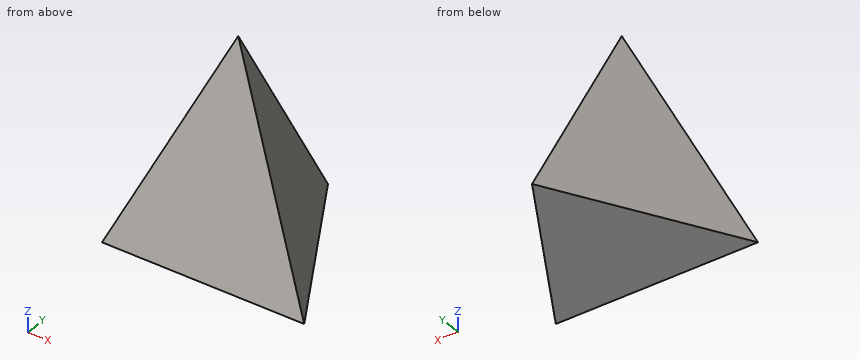
```python
from build123d import *

# Parameters (mm, degrees)
F3_T = -1.524


with BuildPart() as f2:
    # F0 (on Top) → F2 section 0
    with BuildSketch(Plane.XY, mode=Mode.PRIVATE) as f2_s0:
        Polygon((-38.1041381436, -18.5593732185), (38.0958618564, -18.5593732185), (-0.0041380687, 47.4317625066), align=None)
    loft([f2_s0.sketch, Vertex(0, 0, 81.65)])

    # F3 (hollow: no face is removed)
    offset(amount=F3_T, mode=Mode.SUBTRACT)


solid = f2.part
```
Input: part model. Units: mm. Frame: model coordinates. Give positions to 0.01 mm unless a question says otherwise; leave off trailing zeros. Write each loop counter-clockwise with the first axis right and the second up, starting at its lowest first coordinate (ties: lowest second). Pieces come first, ordered by that corner, then holes. Notation, with made-up numbers: (81.5, 81.25) - (120.5, 81.25) arc R21 ccw to (120.5, 117.25) - close; hole circle Ø1 at (24.5, 57.5). An arc over 180 degrees is marked (long way). Write item = value, one per line. Start each with the question number.
1. Section query A-A, the plane x = -12.5. Output: boundary loops of the cut face in (y, z), then the cut area to 3 significant figures.
2. First-contact query: pin 1 Ø10 at (x, z) = (-7, 51.5) entering from +Y; pin 2 Ø5 at (x, z) = (-8.5, 41.5) entering from +Y; pin 3 Ø2 at (x, z) = (-28, 21.5) entering from +Y. Flat tips, straight axial feed; report the tip coordinate or a pass-through.
3. Section query C-C, the plane y = -6. Output: boundary loops of the cut face in (x, z), then the cut area to 3 significant figures.
4. Ray query, L1, parallel to Y at x = 6, z = 17.5; L2, parallel to X at y = 2.5, z = 48.5; L3, parallel to Y at x = -9, z = 8.5. Return the intervals inside material, ascending.
5. Section query B-B, the plane z = 40. Output: boundary loops of the cut face in (x, y), then the cut area to 3 significant figures.
Check sheet entries:
q1.outline = (-18.56, 0) - (25.79, 0) - (-6.09, 54.86) - close; hole (-16.65, 1.52) - (21.73, 1.52) - (-5.86, 49) - close
q1.area = 305 mm2
q2.pin_1 = 14.53
q2.pin_2 = 13.17
q2.pin_3 = -11.72
q3.outline = (-30.85, 0) - (30.84, 0) - (12.32, 55.25) - (-12.32, 55.25) - close; hole (-28.51, 1.52) - (28.5, 1.52) - (12.79, 48.38) - (-12.79, 48.38) - close
q3.area = 450 mm2
q4.L1 = -14.58 to -13.02, 23.69 to 26.87
q4.L2 = -9.68 to -7.84, 7.84 to 9.67
q4.L3 = -16.63 to -15.06, 23.74 to 26.91
q5.outline = (-19.44, -9.47) - (19.43, -9.47) - (0, 24.2) - close; hole (-16.7, -7.9) - (16.7, -7.9) - (0, 21.02) - close
q5.area = 171 mm2
